Input: part model. Units: mm. Frame: model coordinates. A direction names the side the tool comes from. Coordinates: 2 decimals unless noted, no trailing zeros. Loops run counter-clockwise (first coordinate to the right, second up) from the corner with the lowest first, then second, coordinate; pieces in that order, holes last. Notation, with made-up numbers: (36.5, 40) - (53.5, 40) arc R18 ccw to (53.5, 58) - close; hole circle Ø11 at (9, 2.25). An arc over 180 degrees is marked (long way). Answer as CSV lines item,"result". Start each with the question number.
```python
from build123d import *

# Parameters (mm, degrees)
BOSS_EXTRUDE1_DEPTH     = 67.5
CUT_EXTRUDE1_DEPTH      = 243.123064516
CUT_EXTRUDE1_DEPTH_BACK = 243.123064516
SKETCH3_W               = 10
SKETCH3_H               = 10
CUT_EXTRUDE2_DEPTH      = 63
SKETCH13_W              = 105.444668515
SKETCH13_H              = 94.744573391
CUT_EXTRUDE7_DEPTH      = 15
SKETCH7_R               = 1.4
CUT_EXTRUDE3_DEPTH      = 2.5
BOSS_EXTRUDE3_DEPTH     = 2.5
FILLET1_R               = 1
CUT_EXTRUDE4_DEPTH      = 2.5
SKETCH9_R               = 3
SKETCH9_R_2             = 1.4
BOSS_EXTRUDE4_DEPTH     = 4
SKETCH14_W              = 103
SKETCH14_H              = 14.520068356
BOSS_EXTRUDE5_DEPTH     = 2.5
SKETCH15_W              = 100
SKETCH15_H              = 13
BOSS_EXTRUDE6_DEPTH     = 2.5


with BuildPart() as part:
    # Sketch1 → Boss-Extrude1 (new body)
    with BuildSketch(Plane(origin=(0, 0, 0), x_dir=(1, 0, 0), z_dir=(0, 1, 0))):
        Polygon((0, 0), (100, 0), (100, 201.922195993), (97.5, 201.922195993), (2.5, 201.922195993), (2.5, 209.922195993), (0, 209.922195993), (0, 202), (-3, 202), (-3, 92), (0, 92), align=None)
        Polygon((87.5, 199.422195993), (12.5, 199.422195993), (12.5, 189.422195993), (2.5, 189.422195993), (-0.5, 189.422195993), (-0.5, 94.5), (2.5, 94.5), (2.5, 12.5), (12.5, 12.5), (12.5, 2.5), (87.5, 2.5), (87.5, 12.5), (97.5, 12.5), (97.5, 189.422195993), (87.5, 189.422195993), align=None, mode=Mode.SUBTRACT)
    extrude(amount=BOSS_EXTRUDE1_DEPTH)

    # Sketch2 → Cut-Extrude1 (cut, two sides: drawn at the far end of the back side and taken through both)
    with BuildSketch(Plane(origin=(0, 0, 0), x_dir=(0, 0, -1), z_dir=(1, 0, 0)).offset(-CUT_EXTRUDE1_DEPTH_BACK)):
        Polygon((209.922195993, 19.5), (106.520068356, 67.5), (209.922195993, 67.5), align=None)
    extrude(amount=CUT_EXTRUDE1_DEPTH + CUT_EXTRUDE1_DEPTH_BACK, mode=Mode.SUBTRACT)

    # Sketch3 → Cut-Extrude2 (cut)
    with BuildSketch(Plane(origin=(0, 67.5, 0), x_dir=(1, 0, 0), z_dir=(0, 1, 0))):
        with Locations((5, 5)):
            Rectangle(SKETCH3_W, SKETCH3_H)
        with Locations((95, 5)):
            Rectangle(SKETCH3_W, SKETCH3_H)
        with Locations((92.5, 194.422195993)):
            Rectangle(SKETCH3_W, SKETCH3_H)
        with Locations((7.5, 194.422195993)):
            Rectangle(SKETCH3_W, SKETCH3_H)
    extrude(amount=-CUT_EXTRUDE2_DEPTH, mode=Mode.SUBTRACT)

    # Sketch13 → Cut-Extrude7 (cut)
    with BuildSketch(Plane(origin=(0, 67.5, 0), x_dir=(1, 0, 0), z_dir=(0, 1, 0))):
        with Locations((49.722334258, 44.627713304)):
            Rectangle(SKETCH13_W, SKETCH13_H)
    extrude(amount=-CUT_EXTRUDE7_DEPTH, mode=Mode.SUBTRACT)

    # Sketch7 → Cut-Extrude3 (cut)
    with BuildSketch(Plane(origin=(0, 4.5, 0), x_dir=(1, 0, 0), z_dir=(0, 1, 0))):
        with Locations(Location((6.5, 6.5, 0), (0, 0, 270))):
            Circle(SKETCH7_R)
        with Locations(Location((93.5, 6.5, 0), (0, 0, 270))):
            Circle(SKETCH7_R)
        with Locations(Location((93.5, 195.422195993, 0), (0, 0, 270))):
            Circle(SKETCH7_R)
        with Locations(Location((6.5, 195.422195993, 0), (0, 0, 270))):
            Circle(SKETCH7_R)
    extrude(amount=-CUT_EXTRUDE3_DEPTH, mode=Mode.SUBTRACT)

    # Sketch6 → Boss-Extrude3 (add)
    with BuildSketch(Plane(origin=(0, 52.5, 0), x_dir=(1, 0, 0), z_dir=(0, 1, 0))):
        Polygon((0, 10), (10, 10), (10, 0), (90, 0), (90, 10), (100, 10), (100, 92), (0, 92), align=None)
    extrude(amount=BOSS_EXTRUDE3_DEPTH)

    # Fillet1
    fillet1_edges = [part.edges().sort_by_distance(p)[0] for p in [
        (100, 4.5, -5),
        (100, 29.75, -10),
        (95, 4.5, 0),
        (90, 4.5, -5),
        (90, 29.75, 0),
        (95, 4.5, -10),
        (90, 29.75, -10),
        (0, 4.5, -5),
        (5, 4.5, -10),
        (0, 29.75, -10),
        (10, 4.5, -5),
        (10, 29.75, -10),
        (5, 4.5, 0),
        (10, 29.75, 0),
        (5, 55, -10),
        (10, 55, -5),
        (90, 55, -5),
        (95, 55, -10),
    ]]
    fillet(fillet1_edges, radius=FILLET1_R)

    # Sketch8 → Cut-Extrude4 (cut)
    with BuildSketch(Plane(origin=(0, 55, 0), x_dir=(1, 0, 0), z_dir=(0, 1, 0))):
        with BuildLine():
            Line((48, 66.030478743), (48, 69.559887757))
            ThreePointArc((48, 69.559887757), (37.747494154, 64.619743351), (32.751630891, 54.394272549))
            Line((32.751630891, 54.394272549), (36.283905916, 54.394272549))
            ThreePointArc((36.283905916, 54.394272549), (40.222514282, 62.144992148), (48, 66.030478743))
        make_face()
        with BuildLine():
            ThreePointArc((67.250508789, 54.376571097), (62.258779803, 64.613500264), (51.999872379, 69.559902545))
            Line((51.999872379, 69.559902545), (51.995972434, 66.031064817))
            ThreePointArc((51.995972434, 66.031064817), (59.782392543, 62.140116351), (63.718784694, 54.376571097))
            Line((63.718784694, 54.376571097), (67.250508789, 54.376571097))
        make_face()
        with BuildLine():
            ThreePointArc((52.172784101, 35.061770682), (62.371552974, 40.10057205), (67.267297082, 50.368780042))
            Line((67.267297082, 50.368780042), (63.734353685, 50.329807549))
            ThreePointArc((63.734353685, 50.329807549), (59.869305567, 42.547819197), (52.133858688, 38.590446171))
            Line((52.133858688, 38.590446171), (52.172784101, 35.061770682))
        make_face()
        with BuildLine():
            Line((36.256551333, 50.394272549), (32.729870259, 50.394272549))
            ThreePointArc((32.729870259, 50.394272549), (37.744451644, 39.98404241), (48.179365496, 35.021030128))
            Line((48.179365496, 35.021030128), (48.179365496, 38.545347156))
            ThreePointArc((48.179365496, 38.545347156), (40.219436137, 42.45882498), (36.256551333, 50.394272549))
        make_face()
        with BuildLine():
            Line((43.394518847, 50.394272549), (39.801599083, 50.394272549))
            ThreePointArc((39.801599083, 50.394272549), (42.694550048, 44.933492377), (48.179365496, 42.086373682))
            Line((48.179365496, 42.086373682), (48.179365496, 45.670830881))
            ThreePointArc((48.179365496, 45.670830881), (45.170136486, 47.407727524), (43.394518847, 50.394272549))
        make_face()
        with BuildLine():
            Line((48, 58.878040566), (48, 62.480783478))
            ThreePointArc((48, 62.480783478), (42.6977071, 59.670396021), (39.838492389, 54.394272549))
            Line((39.838492389, 54.394272549), (43.451623336, 54.394272549))
            ThreePointArc((43.451623336, 54.394272549), (45.173538583, 57.196387596), (48, 58.878040566))
        make_face()
        with BuildLine():
            ThreePointArc((60.165139128, 54.376571097), (57.30583297, 59.666886795), (51.992050513, 62.482341979))
            Line((51.992050513, 62.482341979), (51.988071163, 58.881655832))
            ThreePointArc((51.988071163, 58.881655832), (54.828637163, 57.194241801), (56.554010489, 54.376571097))
            Line((56.554010489, 54.376571097), (60.165139128, 54.376571097))
        make_face()
        with BuildLine():
            ThreePointArc((52.094713542, 42.139041005), (57.366796475, 44.994838139), (60.178474304, 50.290582046))
            Line((60.178474304, 50.290582046), (56.56234759, 50.250691943))
            ThreePointArc((56.56234759, 50.250691943), (54.863324523, 47.440986584), (52.054994158, 45.739691738))
            Line((52.054994158, 45.739691738), (52.094713542, 42.139041005))
        make_face()
    extrude(amount=-CUT_EXTRUDE4_DEPTH, mode=Mode.SUBTRACT)

    # Sketch9 → Boss-Extrude4 (add)
    # profile 1 of 2: a face of its own
    with BuildSketch(Plane.XZ.offset(-52.5)):
        with Locations(Location((34.040847972, -36.263045043, 0), (0, 0, 90))):
            Circle(SKETCH9_R)
        with Locations(Location((34.040847972, -36.263045043, 0), (0, 0, 270))):
            Circle(SKETCH9_R_2, mode=Mode.SUBTRACT)
    # profile 2 of 2: a face of its own
    with BuildSketch(Plane.XZ.offset(-52.5)):
        with Locations(Location((65.962383475, -68.334497632, 0), (0, 0, 90))):
            Circle(SKETCH9_R)
        with Locations(Location((65.962383475, -68.334497632, 0), (0, 0, 270))):
            Circle(SKETCH9_R_2, mode=Mode.SUBTRACT)
    extrude(amount=BOSS_EXTRUDE4_DEPTH)

    # Sketch14 → Boss-Extrude5 (add)
    with BuildSketch(Plane(origin=(0, 67.5, 0), x_dir=(1, 0, 0), z_dir=(0, 1, 0))):
        with Locations((48.5, 99.260034178)):
            Rectangle(SKETCH14_W, SKETCH14_H)
    extrude(amount=BOSS_EXTRUDE5_DEPTH)

    # Sketch15 → Boss-Extrude6 (add)
    with BuildSketch(Plane.XY.offset(-92)):
        with Locations((50, 61.5)):
            Rectangle(SKETCH15_W, SKETCH15_H)
    extrude(amount=BOSS_EXTRUDE6_DEPTH)


solid = part.part
```
Item 1: Section query C-C, the plane z = -137.5. Output: boundary loops of the cut face in (x, y), and give its area (3 significant figures).
Item 2: Set-up query: faces 4 (the flat face through (52, 11, -201.922)), 5 (the cylindrical face through (45.141, 53.768, -57.164)), 6 (the flat face through (-0.5, 26, -132)), 7 (the flat face through (9, 4.5, -194)). Return all of +Z, -Z, +X, -X, +Y, -Y with unobstructed straight access to the full face (end or side cutting, diameter ignored); none if empty.
Item 3: Contact query for flat-ended pins moving along their axis: P1, Ø11, axis at x = 6, y = 35.5, coming from the -Z side; P2, Ø2, axis at y = 54, z = -43.5, coming from the -X side; P3, Ø6.5, axis at x = 95, z = -3.5, coming from the +Y side. Output: stop coordinate, or through.
Item 4: Draft query along Z for faces 1 (the flat face through (49, 27, 0)), 2 (the flat face through (90, 29, -5)), 3 (the flat face through (87.5, 2, -194)). Return one class per face: pulls with the +Z half, pulls with the -Z half, needs draft (parallel to the pull), parting line crosses it, or undercut.
Item 5: Material intervals for probe 1 along Z at (x, y) = (93.5, 3.1); probe 2 along X at (y, z) = (3.5, -6.5); probe 3 along Z at (x, y) = (30, 6), sorted ascending.
Item 6: Section query A-A, the plane x = 78. Output: boundary loops of the cut face in (y, z), and give its area (3 significant figures).
Response values:
1,outline,"(-3, 0) - (-0.5, 0) - (-0.5, 53.12) - (-3, 53.12) - close; (97.5, 0) - (100, 0) - (100, 53.12) - (97.5, 53.12) - close"
1,area,"266 mm²"
2,face 4,"-Z, +X, +Y, -Y"
2,face 5,"+Y, -Y"
2,face 6,"-Y"
2,face 7,"+Y"
3,P1,"stops at z = -94.5"
3,P2,"stops at x = 0"
3,P3,"stops at y = 4.5"
4,face 1,"pulls with the +Z half"
4,face 2,"needs draft"
4,face 3,"undercut"
5,probe 1,"z = -201.92 to -196.82, -194.02 to -189.42, -12.5 to -7.9, -5.1 to 0"
5,probe 2,"x = 0 to 5.1, 7.9 to 12.5, 87.5 to 92.1, 94.9 to 100"
5,probe 3,"z = -201.92 to -199.42, -2.5 to 0"
6,outline,"(0, -201.92) - (23.21, -201.92) - (24.37, -199.42) - (0, -199.42) - close; (0, -2.5) - (52.5, -2.5) - (52.5, -92) - (67.5, -92) - (67.5, -106.52) - (70, -106.52) - (70, -92) - (68, -92) - (68, -89.5) - (55, -89.5) - (55, 0) - (0, 0) - close"
6,area,"490 mm²"
